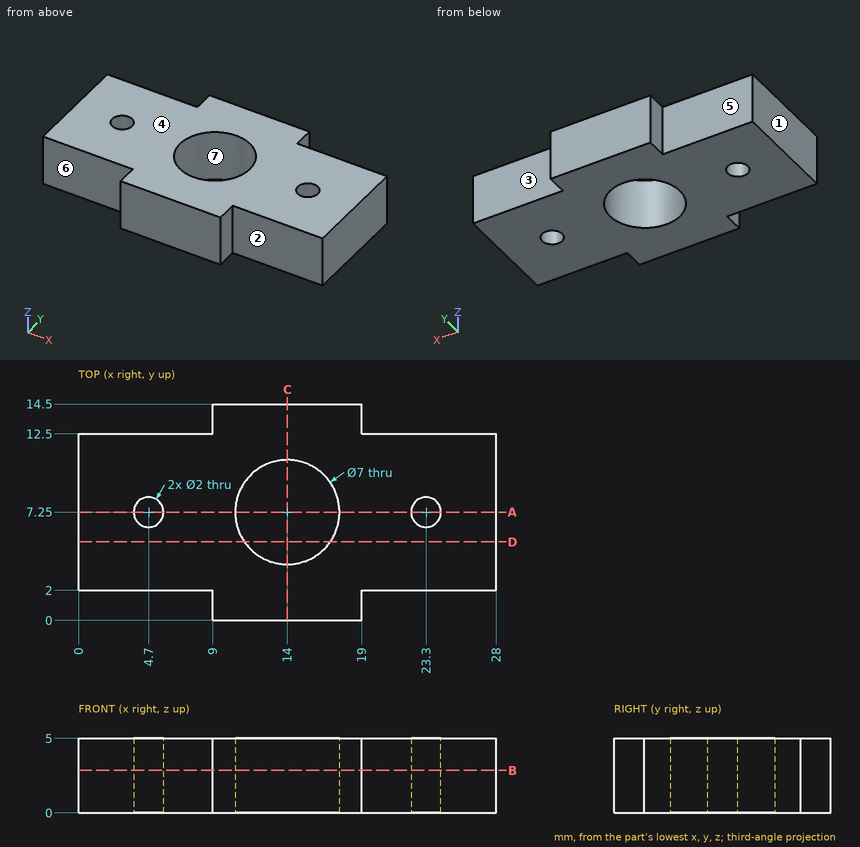
Part print with two shaded views. Sizes in mm from the minimum x, y, z corner. A direction names the side the tool comes from. Round coordinates to 2 decimals unless told otherwise and drop trailing zeros. Order: outer loops, then holes, each group sorted by start corner. A loop starts at its lowest first (then second) coordinate and runs counter-clockwise, first axis right, second up. Notation, with made-up numbers: M 50.25,74.5 L 67.25,74.5 A21 cw 67.25,94.5 Z; hole C 11.5,7.25 d2. An arc over 180 degrees is marked long. Use CSV: the item, a comma, the result in double quotes. Start each with the question number.
(1) Mould opens along Y. For the marked faces 4, 5, 6 and 7 say: +Y half, -Y half, draft (parallel to the pull), parting line (faces both ways), or undercut.
(2) Cut at D-D on y = 5.25. List the corners of the cut face in (x, z), then the cut area to 3 significant figures.
(3) Cut at B-B on z = 2.85. List the corners of the cut face in (x, y).
(4) Cut at C-C on x = 14. List the corners of the cut face in (y, z).
(5) Flat gauge pins, fed straight in: P1, Ø1.2, axis at x = 4.7, y = 7.25, coming from the -Z side; P2, Ø2.5, axis at x = 4.5, z = 3.5, coming from the +Y side; P3, Ø2, axis at y = 0.5, z = 3.5, coming from the -X side; P4, Ø1.6, axis at y = 1.5, z = 3.5, coming from the +X side. Where does each tip first touch, or does it go through?
(6) Tool access for the marked faces 1, 2 and 3: list every direction of +Z, -Z, +X, -X, +Y, -Y with a clear straight run to the whole face (end or side of a thin tool).
(7) Cut at A-A on y = 7.25. List the corners of the cut face in (x, z).
(8) Drill centre lines: probe 1 along Y at (x, z) = (14, 3.55); probe 2 along Y at (x, z) = (4.7, 3.6); probe 3 along X at (y, z) = (9.5, 1.85). Where is each one in solid material? Low to high.
Findings:
1,face 4,"draft"
1,face 5,"+Y half"
1,face 6,"-Y half"
1,face 7,"undercut"
2,outline,"M 0,0 L 11.13,0 L 11.13,5 L 0,5 Z; M 16.87,0 L 28,0 L 28,5 L 16.87,5 Z"
2,area,"111 mm^2"
3,outline,"M 0,2 L 9,2 L 9,0 L 19,0 L 19,2 L 28,2 L 28,12.5 L 19,12.5 L 19,14.5 L 9,14.5 L 9,12.5 L 0,12.5 Z; hole C 4.7,7.25 d2; hole C 14,7.25 d7; hole C 23.3,7.25 d2"
4,outline,"M 0,0 L 3.75,0 L 3.75,5 L 0,5 Z; M 10.75,0 L 14.5,0 L 14.5,5 L 10.75,5 Z"
5,P1,"passes through"
5,P2,"stops at y = 12.5"
5,P3,"stops at x = 9"
5,P4,"stops at x = 28"
6,face 1,"+Z, -Z, -X, +Y, -Y"
6,face 2,"+Z, -Z, +X, -Y"
6,face 3,"+Z, -Z, +X, +Y"
7,outline,"M 0,0 L 3.7,0 L 3.7,5 L 0,5 Z; M 5.7,0 L 10.5,0 L 10.5,5 L 5.7,5 Z; M 17.5,0 L 22.3,0 L 22.3,5 L 17.5,5 Z; M 24.3,0 L 28,0 L 28,5 L 24.3,5 Z"
8,probe 1,"y = 0 to 3.75, 10.75 to 14.5"
8,probe 2,"y = 2 to 6.25, 8.25 to 12.5"
8,probe 3,"x = 0 to 11.32, 16.68 to 28"
